```python
from build123d import *

# Parameters (mm, degrees)
SKETCH2_R           = 1.5
SKETCH2_R_2         = 2.75
BOSS_EXTRUDE1_DEPTH = 2.5


with BuildPart() as part:
    # Sketch2 → Boss-Extrude1 (new body)
    with BuildSketch(Plane(origin=(0, 0, 0), x_dir=(1, 0, 0), z_dir=(0, 1, 0))):
        with BuildLine():
            Line((-20.402989885, -29.497935256), (-19.112268572, -28.051458372))
            ThreePointArc((-19.112268572, -28.051458372), (-17.810696545, -26.629075982), (-16.473919979, -25.239727278))
            ThreePointArc((-16.473919979, -25.239727278), (-14.160863056, -23.377992793), (-11.485697638, -22.089669229))
            ThreePointArc((-11.485697638, -22.089669229), (0, -20.15141071), (11.485697638, -22.089669229))
            ThreePointArc((11.485697638, -22.089669229), (14.160863056, -23.377992793), (16.473919979, -25.239727278))
            ThreePointArc((16.473919979, -25.239727278), (17.810696545, -26.629075982), (19.112268572, -28.051458372))
            Line((19.112268572, -28.051458372), (20.402989885, -29.497935256))
            ThreePointArc((20.402989885, -29.497935256), (35.984508278, -28.676365345), (31.796806607, -13.645668513))
            Line((31.796806607, -13.645668513), (25.794436634, -11.078432427))
            ThreePointArc((25.794436634, -11.078432427), (23.235962273, -9.423067761), (21.376539879, -7.008824278))
            ThreePointArc((21.376539879, -7.008824278), (19.638379202, 0), (21.376539879, 7.008824278))
            ThreePointArc((21.376539879, 7.008824278), (23.235962273, 9.423067761), (25.794436634, 11.078432427))
            Line((25.794436634, 11.078432427), (31.796806607, 13.645668513))
            ThreePointArc((31.796806607, 13.645668513), (35.984508278, 28.676365345), (20.402989885, 29.497935256))
            Line((20.402989885, 29.497935256), (19.112268572, 28.051458372))
            ThreePointArc((19.112268572, 28.051458372), (17.810696545, 26.629075982), (16.473919979, 25.239727278))
            ThreePointArc((16.473919979, 25.239727278), (14.160863056, 23.377992793), (11.485697638, 22.089669229))
            ThreePointArc((11.485697638, 22.089669229), (0, 20.15141071), (-11.485697638, 22.089669229))
            ThreePointArc((-11.485697638, 22.089669229), (-14.160863056, 23.377992793), (-16.473919979, 25.239727278))
            ThreePointArc((-16.473919979, 25.239727278), (-17.810696545, 26.629075982), (-19.112268572, 28.051458372))
            Line((-19.112268572, 28.051458372), (-20.402989885, 29.497935256))
            ThreePointArc((-20.402989885, 29.497935256), (-35.984508278, 28.676365345), (-31.796806607, 13.645668513))
            Line((-31.796806607, 13.645668513), (-25.794436634, 11.078432427))
            ThreePointArc((-25.794436634, 11.078432427), (-23.235962273, 9.423067761), (-21.376539879, 7.008824278))
            ThreePointArc((-21.376539879, 7.008824278), (-19.638379202, 0), (-21.376539879, -7.008824278))
            ThreePointArc((-21.376539879, -7.008824278), (-23.235962273, -9.423067761), (-25.794436634, -11.078432427))
            Line((-25.794436634, -11.078432427), (-31.796806607, -13.645668513))
            ThreePointArc((-31.796806607, -13.645668513), (-35.984508278, -28.676365345), (-20.402989885, -29.497935256))
        make_face()
        with Locations(Location((15.365, -15.365, 0), (0, 0, 270))):
            Circle(SKETCH2_R, mode=Mode.SUBTRACT)
        with Locations(Location((27.864354565, 22.840004863, 0), (0, 0, 270))):
            Circle(SKETCH2_R_2, mode=Mode.SUBTRACT)
        with Locations(Location((-15.365, 15.365, 0), (0, 0, 270))):
            Circle(SKETCH2_R, mode=Mode.SUBTRACT)
        with Locations(Location((15.365, 15.365, 0), (0, 0, 270))):
            Circle(SKETCH2_R, mode=Mode.SUBTRACT)
        with Locations(Location((-15.365, -15.365, 0), (0, 0, 270))):
            Circle(SKETCH2_R, mode=Mode.SUBTRACT)
        with Locations(Location((27.864354565, -22.840004863, 0), (0, 0, 270))):
            Circle(SKETCH2_R_2, mode=Mode.SUBTRACT)
        with Locations(Location((10.000016395, -10.000011804, 0), (0, 0, 270))):
            Circle(SKETCH2_R_2, mode=Mode.SUBTRACT)
        with Locations(Location((-27.864354565, 22.840004863, 0), (0, 0, 270))):
            Circle(SKETCH2_R_2, mode=Mode.SUBTRACT)
        with Locations(Location((-27.864354565, -22.840004863, 0), (0, 0, 270))):
            Circle(SKETCH2_R_2, mode=Mode.SUBTRACT)
        with Locations(Location((-10.000016395, -10.000011804, 0), (0, 0, 270))):
            Circle(SKETCH2_R_2, mode=Mode.SUBTRACT)
        with Locations(Location((-10.000016395, 10.000011804, 0), (0, 0, 270))):
            Circle(SKETCH2_R_2, mode=Mode.SUBTRACT)
        with Locations(Location((10.000016395, 10.000011804, 0), (0, 0, 270))):
            Circle(SKETCH2_R_2, mode=Mode.SUBTRACT)
        with BuildLine():
            Line((3.71054333, -12.635244665), (0.769622246, -9.090373716))
            ThreePointArc((0.769622246, -9.090373716), (0, -8.728873205), (-0.769622246, -9.090373716))
            Line((-0.769622246, -9.090373716), (-3.71054333, -12.635244665))
            ThreePointArc((-3.71054333, -12.635244665), (-3.829359507, -13.73273998), (-2.865512851, -14.2708969))
            ThreePointArc((-2.865512851, -14.2708969), (0, -14.16270124), (2.865512851, -14.2708969))
            ThreePointArc((2.865512851, -14.2708969), (3.829359508, -13.73273998), (3.71054333, -12.635244665))
        make_face(mode=Mode.SUBTRACT)
        with BuildLine():
            Line((-3.71054333, 12.635244665), (-0.769622246, 9.090373716))
            ThreePointArc((-0.769622246, 9.090373716), (0, 8.728873205), (0.769622246, 9.090373716))
            Line((0.769622246, 9.090373716), (3.71054333, 12.635244665))
            ThreePointArc((3.71054333, 12.635244665), (3.829359507, 13.73273998), (2.865512851, 14.2708969))
            ThreePointArc((2.865512851, 14.2708969), (0, 14.16270124), (-2.865512851, 14.2708969))
            ThreePointArc((-2.865512851, 14.2708969), (-3.829359508, 13.73273998), (-3.71054333, 12.635244665))
        make_face(mode=Mode.SUBTRACT)
    extrude(amount=BOSS_EXTRUDE1_DEPTH)


solid = part.part
```
For this review, take the finished solid that the model builds, in its own axes (mm). A direction names the side the tool comes from. Coordinates: 2 decimals unless noted, no trailing zeros. Loops run counter-clockwise (first coordinate to the right, second up) from the corner with the lowest first, then second, coordinate; pieces in that order, holes last. Notation, with made-up numbers: (53, 44) -> (104, 44) arc R34 cw to (104, 74) -> close; hole circle Ø9 at (-12, 83). An arc over 180 degrees is marked (long way). Return JSON: item names as keys, results as strings. Group by question number.
(1) Consider section D-D, the plane z = -0.5. Give the boundary of the cut face in (x, y).
(2) Consider section A-A, the plane z = -10. Give the boundary of the cut face in (x, y), plus the area to 3 significant figures.
(3) To check wall thickness, follow L1, parallel to X at y = 0.6, z = -14; L2, parallel to X at y = 0.2, z = -22.5; L3, parallel to X at y = 1.6, z = -16.5. State the ranges of each line that lie inside material, in increasing order.
(4) Consider section C-C, the plane y = 1. Count the separate pieces of the cut face and the enclosed holes in it, plus the area to 3 significant figures.
(5) Tool access review of faces 5 (the flat face through (-28.754, 1.232, 12.344)), 6 (the flat face through (28.84, 1.23, 12.38)), 7 (the cylindrical face through (14.13, 1.23, 23.36)), 8 (the flat face through (2.22, 1.23, -10.84)), 9 (the cylindrical face through (0.16, 1.23, -20.15)): name each direction out of +Z, -Z, +X, -X, +Y, -Y from which nothing blocks a thin tool from reaching the whole face with its end or side.
(6) For pin 1 Ø5 at (x, z) = (27.86, -22.84) entering from +Y, flat-tipped, find the tip position at first contact; note if it passes through.
(7) Consider section B-B, the plane x = 27. Give the boundary of the cut face in (y, z), plus the area to 3 significant figures.
(8) Mouldability with a two-part tool opening along Z and no side actions: class faces 1 (the cylindrical face through (-17.792, 1.232, -26.609)), 2 (the flat face through (28.754, 1.232, -12.344)), 3 (the cylindrical face through (-19.64, 1.23, -0.1)), 4 (the cylindrical face through (17.792, 1.232, 26.609)) as pulls with the +Z half, pulls with the -Z half, needs draft (parallel to the pull), parting line crosses it, or undercut.
Results below:
{
 "1": {"outline": "(-19.65, 0) -> (19.65, 0) -> (19.65, 2.5) -> (-19.65, 2.5) -> close"},
 "2": {"outline": "(-23.93, 0) -> (-12.75, 0) -> (-12.75, 2.5) -> (-23.93, 2.5) -> close; (-7.25, 0) -> (-1.52, 0) -> (-1.52, 2.5) -> (-7.25, 2.5) -> close; (1.52, 0) -> (7.25, 0) -> (7.25, 2.5) -> (1.52, 2.5) -> close; (12.75, 0) -> (23.93, 0) -> (23.93, 2.5) -> (12.75, 2.5) -> close", "area": "84.5 mm2"},
 "3": {"L1": "x = -32.54 to -15.99, -14.74 to -3.63, 3.63 to 14.74, 15.99 to 32.54", "L2": "x = -37.86 to -30.59, -25.14 to -12.52, 12.52 to 25.14, 30.59 to 37.86", "L3": "x = -35.6 to -16.35, -14.38 to 14.38, 16.35 to 35.6"},
 "4": {"separate pieces": "1", "enclosed holes": "14", "area": "2,860 mm2"},
 "5": {"face 5": "-X, +Y, -Y", "face 6": "+X, +Y, -Y", "face 7": "+Z, +Y, -Y", "face 8": "+Y, -Y", "face 9": "-Z, +Y, -Y"},
 "6": {"pin 1": "passes through"},
 "7": {"outline": "(0, -32.8) -> (2.5, -32.8) -> (2.5, -25.45) -> (0, -25.45) -> close; (0, -20.23) -> (2.5, -20.23) -> (2.5, -11.59) -> (0, -11.59) -> close; (0, 11.59) -> (2.5, 11.59) -> (2.5, 20.23) -> (0, 20.23) -> close; (0, 25.45) -> (2.5, 25.45) -> (2.5, 32.8) -> (0, 32.8) -> close", "area": "79.9 mm2"},
 "8": {"face 1": "pulls with the -Z half", "face 2": "undercut", "face 3": "undercut", "face 4": "pulls with the +Z half"}
}
